Design review of the part built by this model. Coordinates are the model's own, in mm. Face numbers are marked on the shaded views. A direction names the side the tool comes from. Give positions to 0.01 mm unless a question says otherwise; leave off trailing zeros. Order: outer loops, then holes, each group sorted by start corner. A loop starts at its lowest first (then second) coordinate and runs counter-clockwise, first axis right, second up. Notation, with made-up numbers: (60, 49.25) -> (105, 49.25) arc R11 cw to (105, 56.25) -> close; hole circle Ø10 at (65, 88). An arc over 180 degrees is marked (long way). Use a Markdown table: item, result. Add a question column.
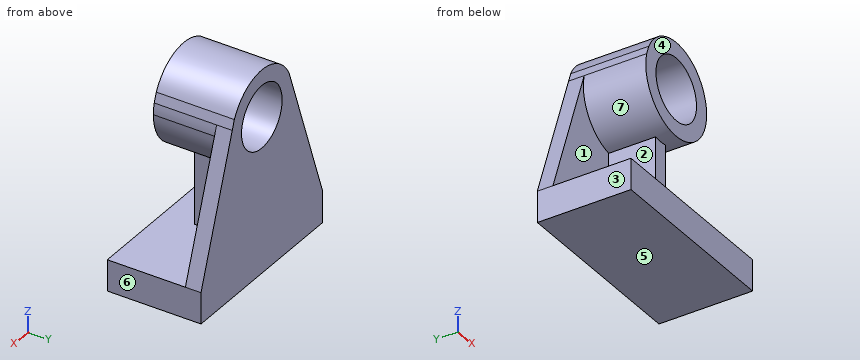
```python
from build123d import *

# Parameters (mm, degrees)
F1_DEPTH = 25.4
F0_W     = 304.8
F0_H     = 50.8
F2_DEPTH = 152.4
F0_R     = 50.8
F3_DEPTH = 127
F4_W     = 76.2
F4_H     = 139.571316
F5_DEPTH = 12.7


with BuildPart() as f1:
    # F0 (on Front) → F1 (new body)
    with BuildSketch(Plane.XZ):
        with BuildLine():
            Line((-74.069707, 34.275554), (-152.4, -186.816301))
            Line((-152.4, -186.816301), (152.4, -186.816301))
            Line((152.4, -186.816301), (74.069707, 34.275554))
            ThreePointArc((74.069707, 34.275554), (75.665553, 25.392814), (76.2, 16.383699))
            ThreePointArc((76.2, 16.383699), (-9.009115, -59.281853), (-74.069707, 34.275554))
        make_face()
    extrude(amount=F1_DEPTH)

    # F0 (on Front) → F2 (join)
    with BuildSketch(Plane.XZ):
        with Locations((0, -212.216301)):
            Rectangle(F0_W, F0_H)
    extrude(amount=F2_DEPTH)

    # F0 (on Front) → F3 (join)
    with BuildSketch(Plane.XZ):
        with BuildLine():
            Line((-68.812805, 49.11347), (-74.069707, 34.275554))
            ThreePointArc((-74.069707, 34.275554), (-9.009115, -59.281853), (76.2, 16.383699))
            ThreePointArc((76.2, 16.383699), (75.665553, 25.392814), (74.069707, 34.275554))
            Line((74.069707, 34.275554), (68.812805, 49.11347))
            ThreePointArc((68.812805, 49.11347), (0, 92.583699), (-68.812805, 49.11347))
        make_face()
        with Locations((0, 16.383699)):
            Circle(F0_R, mode=Mode.SUBTRACT)
    extrude(amount=F3_DEPTH)

    # F4 (on Right) → F5 (join, symmetric)
    with BuildSketch(Plane.YZ):
        with Locations((-63.5, -117.019369)):
            Rectangle(F4_W, F4_H)
    extrude(amount=F5_DEPTH, both=True)


solid = f1.part
```
1) Add section A-A (y = -33). Give the boundary of the cut face in (x, z), then the cut area to 3 significant figures.
2) For L1, parallel to Z at x = 1, y = -24; L2, parallel to Z at x = 40, y = -32.5; L3, parallel to Y at x = -28, z = -54, list the stretches that pass through material, from the lowest coordinate up. Write a range as [from, to].
3) The part is to be moulded in two halves that separate along Z. For the marked faces 5, 6 and 7, say which applies: +Z half, -Z half, draft (parallel to the pull), parting line (faces both ways), or undercut.
4) Insertion check: pin 1 (10 mm diameter, centred on x = 25.5, z = -16.5, fed in from -Y); pin 2 (3 mm diameter, centred on y = -52.5, z = -158.5, fed in from +X); pin 3 (1 mm diameter, centred on x = 6.5, z = -153.5, fed in from -Y); pin 4 (4 mm diameter, centred on x = 42.5, y = -45, fed in from +Z). Each pin has a flat end and moves straight along its axis. Give the tip position at first contact, or say it passes through.
5) Add section C-C (z = 25). Give the boundary of the cut face in (x, y).
6) Add section D-D (y = -120). Give the boundary of the cut face in (x, z).
7) Machinability: for the marked faces 1, 2, 3 and 4, which of the approach directions +Z, -Z, +X, -X, +Y, -Y give a long, thin tool a straight path to every point of the face, cutting with its end or side? Answer none if there is none.
Worked answers:
| question | item | result |
|---|---|---|
| 1 | outline | (-152.4, -237.62) -> (152.4, -237.62) -> (152.4, -186.82) -> (-152.4, -186.82) -> close; (-74.07, 34.28) arc R76.2 ccw to (-12.7, -58.75) -> (-12.7, -186.81) -> (12.7, -186.81) -> (12.7, -58.75) arc R76.2 ccw to (76.2, 16.38) arc R76.2 ccw to (74.07, 34.28) -> (68.81, 49.11) arc R76.2 ccw to (-68.81, 49.11) -> close; hole circle Ø101.6 at (0, 16.38) |
| 1 | area | 28,800 mm^2 |
| 2 | L1 | [-237.62, -34.41], [67.17, 92.58] |
| 2 | L2 | [-237.62, -186.82], [-48.47, -14.93], [47.7, 81.24] |
| 2 | L3 | [-127, 0] |
| 3 | face 5 | -Z half |
| 3 | face 6 | draft |
| 3 | face 7 | undercut |
| 4 | pin 1 | through |
| 4 | pin 2 | x = 12.7 |
| 4 | pin 3 | y = -101.6 |
| 4 | pin 4 | z = 80.93 |
| 5 | outline | (-77.36, -25.4) -> (-75.71, -25.4) -> (-75.71, -127) -> (-50.06, -127) -> (-50.06, 0) -> (-77.36, 0) -> close; (50.06, -127) -> (75.71, -127) -> (75.71, -25.4) -> (77.36, -25.4) -> (77.36, 0) -> (50.06, 0) -> close |
| 6 | outline | (-152.4, -237.62) -> (152.4, -237.62) -> (152.4, -186.82) -> (-152.4, -186.82) -> close; (-74.07, 34.28) arc R76.2 ccw (long way) to (76.2, 16.38) arc R76.2 ccw to (74.07, 34.28) -> (68.81, 49.11) arc R76.2 ccw to (-68.81, 49.11) -> close; hole circle Ø101.6 at (0, 16.38) |
| 7 | face 1 | -Y |
| 7 | face 2 | -X, -Y |
| 7 | face 3 | +Z, -Z, -X, +Y, -Y |
| 7 | face 4 | +Z, +X, -X, -Y |
